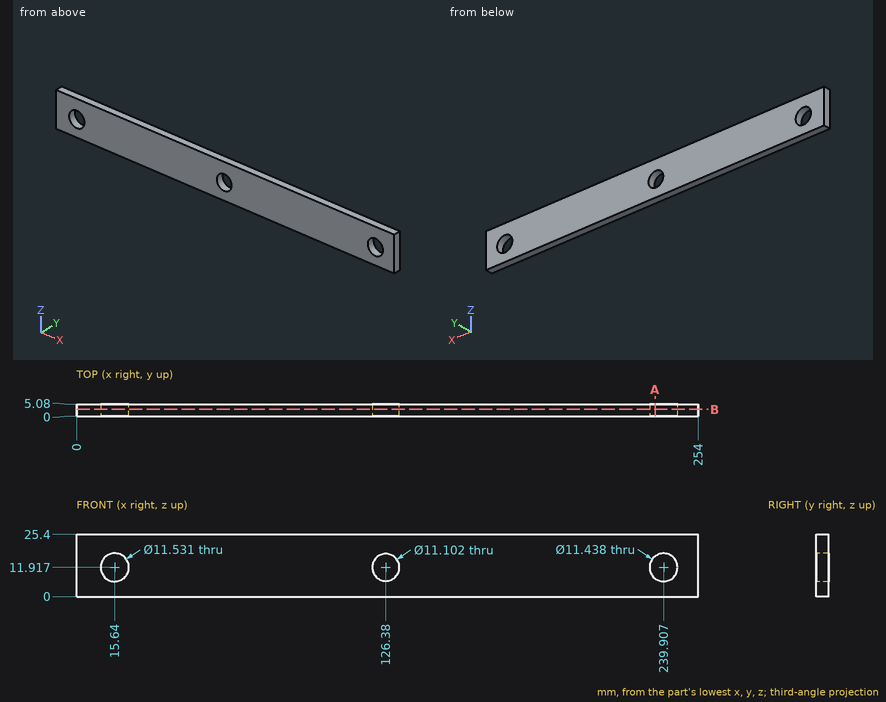
Answer from the drawing. Dimensions are ordinates in mm from the lowest x, y and z of the part. Give positions to 0.01 mm unless a question says otherwise; leave off trailing zeros. Order: outer loops, then holes, each group sorted by start corner. A loop starts at its lowest first (then second) coordinate and runs counter-clockwise, first axis right, second up. Notation, with made-up numbers: (86.5, 25.5) - (128.5, 25.5) arc R32 cw to (128.5, 53.5) - close; hole circle Ø6 at (76.5, -4.75). An arc over 180 degrees is marked (long way). One line per item, written item: value. Start each with the question number.
1. This flat-tipped pin is pushed along its axis until it touches: pin 1 Ø14.5 at (x, z) = (126.38, 11.92) entering from +Y. Where does it stop, or does it pass through?
2. Section A-A, the plane x = 236.5 is taken. Write down the section's boundary in (y, z).
3. Consider line 1 (X direction, y = 0.35, z = 11.75); line 2 (X direction, y = 4.3, z = 9.5) (1 decimal); line 3 (Z direction, x = 17, y = 3.1) (1 decimal). Determine where each line is inside the solid, lowest interval first.
4. Section B-B, the plane y = 2.9 is taken. Write down the section's boundary in (x, z) (1 decimal), then the cut area to 3 significant figures.
Filled sheet:
1. pin 1: y = 5.08
2. outline: (0, 0) - (5.08, 0) - (5.08, 7.32) - (0, 7.32) - close; (0, 16.51) - (5.08, 16.51) - (5.08, 25.4) - (0, 25.4) - close
3. line 1: 0 to 9.88, 21.4 to 120.83, 131.93 to 234.19, 245.62 to 254
3. line 2: 0 to 10.4, 20.9 to 121.4, 131.4 to 234.7, 245.1 to 254
3. line 3: 0 to 6.3, 17.5 to 25.4
4. outline: (0, 0) - (254, 0) - (254, 25.4) - (0, 25.4) - close; hole circle Ø11.5 at (15.6, 11.9); hole circle Ø11.1 at (126.4, 11.9); hole circle Ø11.4 at (239.9, 11.9)
4. area: 6,150 mm²
